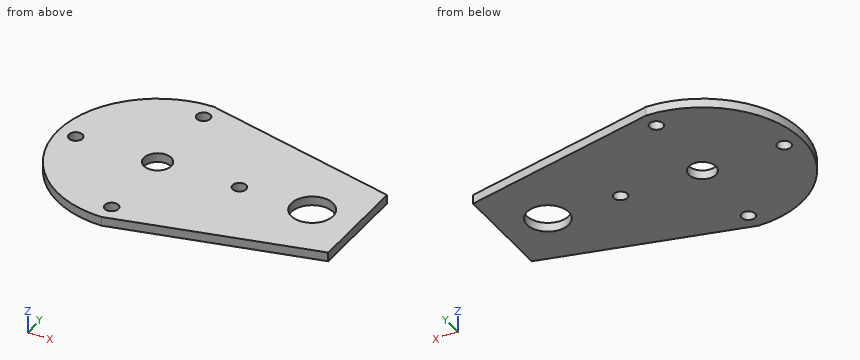
from build123d import *

# Parameters (mm, degrees)
SKETCH_1_R      = 1.5
SKETCH_1_R_2    = 3
SKETCH_1_R_3    = 4.6
EXTRUDE_1_DEPTH = 2


with BuildPart() as part:
    # 草图1 → 凸台-拉伸1 (new body)
    with BuildSketch(Plane.XY):
        with BuildLine():
            Line((5.001004832, -11.501004832), (5.001004832, 11.501004832))
            Line((5.001004832, 11.501004832), (-38.998995168, 22.002009663))
            ThreePointArc((-38.998995168, 22.002009663), (-61.001004832, 0), (-38.998995168, -22.002009663))
            Line((-38.998995168, -22.002009663), (5.001004832, -11.501004832))
        make_face()
        with Locations((-38.998995168, -18.002009663)):
            Circle(SKETCH_1_R, mode=Mode.SUBTRACT)
        with Locations((-57.001004832, 0)):
            Circle(SKETCH_1_R, mode=Mode.SUBTRACT)
        with Locations((-38.998995168, 0)):
            Circle(SKETCH_1_R_2, mode=Mode.SUBTRACT)
        with Locations((-38.998995168, 18.002009663)):
            Circle(SKETCH_1_R, mode=Mode.SUBTRACT)
        with Locations((-20.996985505, 0)):
            Circle(SKETCH_1_R, mode=Mode.SUBTRACT)
        with Locations((-4.998995168, 0)):
            Circle(SKETCH_1_R_3, mode=Mode.SUBTRACT)
    extrude(amount=EXTRUDE_1_DEPTH)


solid = part.part
Could you check a few things on this model? Use its own coordinates, in mm. Coordinates: 2 decimals unless noted, no trailing zeros. Loops run counter-clockwise (first coordinate to the right, second up) from the corner with the lowest first, then second, coordinate; pieces in that order, holes last.
1. Imagine slicing it at A-A (y = 0). Please give me the cut outline in (x, z).
2. Imagine slicing it at C-C (z = 1.45). Please give me the cut outline in (x, y).
3. Imagine slicing it at B-B (x = -2). Please give me the cut outline in (y, z), and give its area (3 significant figures).
4. Imagine slicing it at D-D (y = -14). Please give me the cut outline in (x, z), and give its area (3 significant figures).
5. I need wall thicknesses on L1, parallel to X at y = -2, z = 0.2; L2, parallel to Y at x = -38.5, z = 1.3; L3, parallel to Y at x = -5.5, z = 0.5. Which ranges of each line are inside material? Lowest first, please.
6. For P1, Ø3.5, axis at x = -57, y = 0, coming from the +Z side, with a flat end and sliding along its axis, tell me the tip position at first contact or that it passes through.
Computed values:
1. outline: (-61, 0) - (-58.5, 0) - (-58.5, 2) - (-61, 2) - close; (-55.5, 0) - (-42, 0) - (-42, 2) - (-55.5, 2) - close; (-36, 0) - (-22.5, 0) - (-22.5, 2) - (-36, 2) - close; (-19.5, 0) - (-9.6, 0) - (-9.6, 2) - (-19.5, 2) - close; (-0.4, 0) - (5, 0) - (5, 2) - (-0.4, 2) - close
2. outline: (-39, -22) - (5, -11.5) - (5, 11.5) - (-39, 22) arc R22 ccw to start; hole circle Ø3 at (-57, 0); hole circle Ø6 at (-39, 0); hole circle Ø3 at (-39, -18); hole circle Ø3 at (-39, 18); hole circle Ø3 at (-21, 0); hole circle Ø9.2 at (-5, 0)
3. outline: (-13.17, 0) - (-3.49, 0) - (-3.49, 2) - (-13.17, 2) - close; (3.49, 0) - (13.17, 0) - (13.17, 2) - (3.49, 2) - close
3. area: 38.7 mm2
4. outline: (-55.97, 0) - (-5.47, 0) - (-5.47, 2) - (-55.97, 2) - close
4. area: 101 mm2
5. L1: x = -60.91 to -41.24, -36.76 to -9.14, -0.86 to 5
5. L2: y = -21.88 to -19.42, -16.59 to -2.96, 2.96 to 16.59, 19.42 to 21.88
5. L3: y = -14.01 to -4.57, 4.57 to 14.01
6. P1: stops at z = 2
